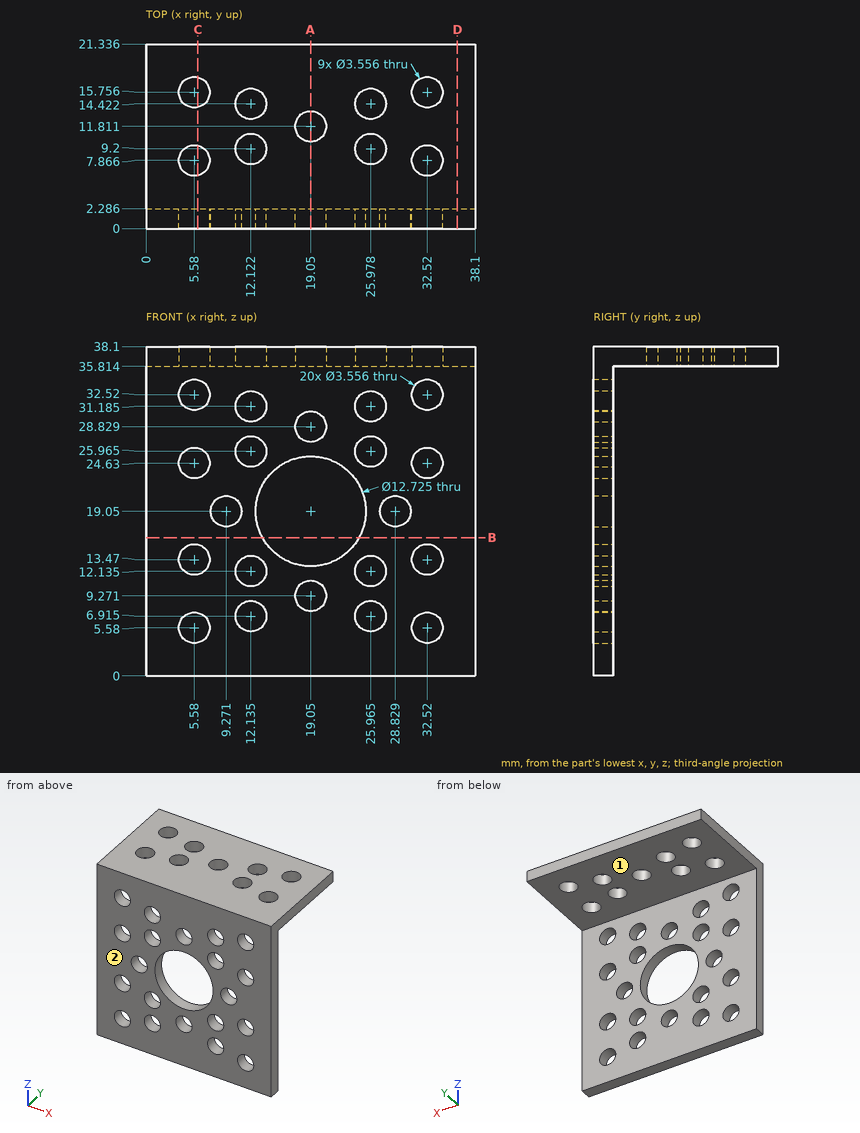
Verification items for this drawing (mm, ordinates from the low corner). A direction names the side the tool comes from. Give positions to 0.01 mm unless a question says otherwise; leave off trailing zeros. Write each loop counter-clockwise with the first axis right and the second up, starting at its lowest first coordinate (ties: lowest second). Pieces come first, ordered by that corner, then holes. Notation, with made-up numbers: (-24.5, 12) -> (5.5, 12) arc R17 cw to (5.5, 44) -> close; hole circle Ø5 at (-35.75, 19.5). An arc over 180 degrees is marked (long way). Use one line per item in the form item = value.
Item 1: Access from +Z, -Z, +X, -X, +Y, -Y to the whole of each face (thin tool, end or side, straight path). Record for the marked faces 1 and 2.
Results list:
face_1 = -Z, +X, -X, +Y
face_2 = +Z, -Z, +X, -X, -Y
Item 2: Sectioned sample at A-A on x = 19.05. Enter the section's corners in (y, z).
Results list:
outline = (0, 0) -> (2.29, 0) -> (2.29, 7.49) -> (0, 7.49) -> close; (0, 11.05) -> (2.29, 11.05) -> (2.29, 12.69) -> (0, 12.69) -> close; (0, 25.41) -> (2.29, 25.41) -> (2.29, 27.05) -> (0, 27.05) -> close; (0, 30.61) -> (2.29, 30.61) -> (2.29, 35.81) -> (10.03, 35.81) -> (10.03, 38.1) -> (0, 38.1) -> close; (13.59, 35.81) -> (21.34, 35.81) -> (21.34, 38.1) -> (13.59, 38.1) -> close
Item 3: Sectioned sample at C-C on x = 6. Count the separate pieces of the cut face and the enclosed holes in it.
Results list:
separate_pieces = 7
enclosed_holes = 0
Item 4: Sectioned sample at D-D on x = 36. Enter the section's corners in (y, z), plus the area to 3 significant figures.
Results list:
outline = (0, 0) -> (2.29, 0) -> (2.29, 35.81) -> (21.34, 35.81) -> (21.34, 38.1) -> (0, 38.1) -> close
area = 131 mm2
Item 5: Scan lines: line 1 (X direction, y = 1.4, z = 19.05); line 2 (X direction, y = 1.75, z = 19.5); line 3 (Y direction, x = 31, z = 12.5). Record each from-to range of solid material in increasing order.
Results list:
line_1 = 0 to 7.49, 11.05 to 12.69, 25.41 to 27.05, 30.61 to 38.1
line_2 = 0 to 7.55, 10.99 to 12.7, 25.4 to 27.11, 30.55 to 38.1
line_3 = 0 to 2.29
Item 6: Depth check by flat-ended pin: pin 1 Ø1 at (x, z) = (28, 27.5) entering from +Y; pin 2 Ø12 at (x, y) = (32.5, 10.5) entering from -Z. Enter the tip coordinate at first touch or a pass-through.
Results list:
pin_1 = 2.29
pin_2 = 35.81
Item 7: Sectioned sample at B-B on z = 16. Enter the section's corners in (x, y).
Results list:
outline = (0, 0) -> (13.47, 0) -> (13.47, 2.29) -> (0, 2.29) -> close; (24.63, 0) -> (38.1, 0) -> (38.1, 2.29) -> (24.63, 2.29) -> close
